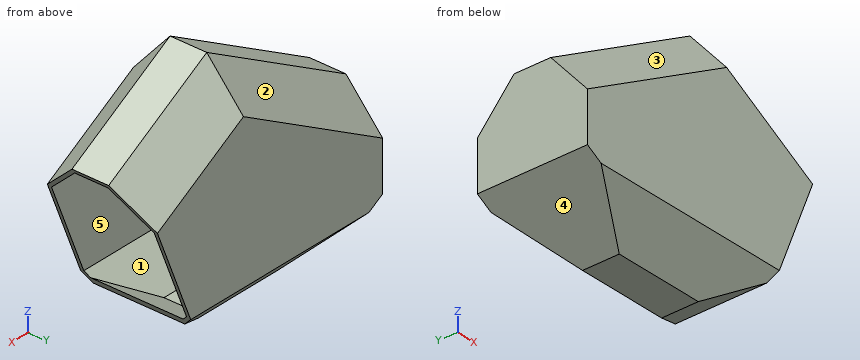
```python
from build123d import *

# Parameters (mm, degrees)
F1_DEPTH = 30
F2_SIZE  = 20
F3_T     = -2


with BuildPart() as f1:
    # F0 (on Front) → F1 (new body, symmetric)
    with BuildSketch(Plane.XZ):
        Polygon((0, 25), (0, -25), (43.3012701892, -50), (93.3012701892, -50), (119.2820323028, -35), (150, 40), (87.9903810568, 75.8012701892), align=None)
    extrude(amount=F1_DEPTH, both=True)

    # F2
    f2_edges = [f1.edges().sort_by_distance(p)[0] for p in [
        (68.30127, -30, -50),
        (68.30127, 30, -50),
        (43.995191, -30, 50.400635),
        (118.995191, -30, 57.900635),
        (118.995191, 30, 57.900635),
        (43.995191, 30, 50.400635),
    ]]
    chamfer(f2_edges, length=F2_SIZE)

    # F3
    f3_openings = [f1.faces().sort_by_distance(p)[0] for p in [
        (133.563862, 0, -0.129945),
    ]]
    offset(amount=F3_T, openings=f3_openings)


solid = f1.part
```
Can you work these out from the model? Positions are in its coordinate system, mm. Face numbers are marked on the shaded views. A direction names the side the tool comes from. Give positions to 0.01 mm unless a question says otherwise; leave off trailing zeros. Order: outer loops, then holes, each group sorted by start corner. A loop starts at its lowest first (then second) coordinate and runs counter-clockwise, first axis right, second up. Notation, with made-up numbers: (-29, 80.25) - (23, 80.25) arc R27 ccw to (23, 104.25) - close; hole circle Ø8 at (68.5, 18.5). An arc over 180 degrees is marked (long way). Use a Markdown table: item, result. Add a question column.
Q1. If we section it at C-C on y = -17.5: Write out the boundary of the cut face in (x, z).
Q2. If we section it at B-B on z = 58: Write out the boundary of the cut face in (x, y).
Q3. I'm going to push flat-ended pins straight in: pin 1 (4 mm diameter, centred on x = 51.5, y = 13, fed in from +Z); pin 2 (3 mm diameter, centred on y = -7, z = -28.5, fed in from +X); pin 3 (4 mm diameter, centred on x = 37, y = -11, fed in from -Z). Where does each tip first touch, or does it pass through?
Q4. Please list where these lines run through material, in increasing order: line 1 along Y through (x, z) = (63, 24); line 2 along X through (y, z) = (16, -10); line 3 along Z through (x, y) = (88, -20).
Q5. If we mould it in two halves opening along Y, with no side actions, what happens to the marked faces 1, 2 and 3? For each: released by +Y, released by -Y, zero draft, split by the parting line, or undercut.
Q6. If we section it at A-A on x = 38: Write out the boundary of the cut face in (y, z).
Q7. If we section it at D-D on z = 30: Write out the boundary of the cut face in (x, y).
Q8. On a 3-axis mill with a long thin cutter (end or side, diameter ignored), from which of +Z, -Z, +X, -X, +Y, -Y can I reach the whole of each face in a straight line? I mean the marked faces 4 and 5. Say none if no direction works.
Answers follow:
| question | item | result |
|---|---|---|
| 1 | outline | (0, -25) - (30.31, -42.5) - (106.29, -42.5) - (119.28, -35) - (120.52, -31.98) - (107.19, -39.67) - (29.41, -39.67) - (2, -23.85) - (2, 14.23) - (87.99, 63.88) - (146.05, 30.35) - (147.13, 33) - (87.99, 67.14) - (0, 16.34) - close |
| 2 | outline | (57.16, -10) - (87.99, -25.42) - (118.82, -10) - (118.82, 10) - (87.99, 25.42) - (57.16, 10) - close; hole (61.16, -9.17) - (87.99, -22.59) - (114.82, -9.17) - (114.82, 9.17) - (87.99, 22.59) - (61.16, 9.17) - close |
| 3 | pin 1 | stops at z = 53.85 |
| 3 | pin 2 | stops at x = 12.66 |
| 3 | pin 3 | stops at z = -47.52 |
| 4 | line 1 | y = -30 to -28, 28 to 30 |
| 4 | line 2 | x = 0 to 2 |
| 4 | line 3 | z = -40 to -37.17, 60.98 to 64.25 |
| 5 | face 1 | undercut |
| 5 | face 2 | released by +Y |
| 5 | face 3 | released by -Y |
| 6 | outline | (-30, -30) - (-13.06, -46.94) - (13.06, -46.94) - (30, -30) - (30, 23.85) - (10, 46.94) - (-10, 46.94) - (-30, 23.85) - close; hole (-28, -29.17) - (-12.54, -44.63) - (12.54, -44.63) - (28, -29.17) - (28, 22.89) - (9.17, 44.63) - (-9.17, 44.63) - (-28, 22.89) - close |
| 7 | outline | (8.66, -10) - (48.66, -30) - (127.32, -30) - (145.9, -20.71) - (145.9, -17.88) - (125.66, -28) - (50.32, -28) - (12.66, -9.17) - (12.66, 9.17) - (50.32, 28) - (125.66, 28) - (145.9, 17.88) - (145.9, 20.71) - (127.32, 30) - (48.66, 30) - (8.66, 10) - close |
| 8 | face 4 | -Z, -X, +Y, -Y |
| 8 | face 5 | none |
